```python
from build123d import *

# Parameters (mm, degrees)
SKETCH1_W          = 58
SKETCH1_H          = 34
EXTRUDE1_DEPTH     = 1.6
SKETCH2_W          = 38
SKETCH2_H          = 6
EXTRUDE2_DEPTH     = 8.5
SKETCH3_W          = 9
SKETCH3_H          = 33
EXTRUDE3_DEPTH     = 9.2
SKETCH4_W          = 16.4
SKETCH4_H          = 12.2
EXTRUDE4_DEPTH     = 11
CUT_EXTRUDE1_DEPTH = 14
FILLET1_R          = 1
FILLET2_R          = 0.5


with BuildPart() as part:
    # Sketch1 → Extrude1 (new body)
    with BuildSketch(Plane.XY):
        with Locations((29, 17)):
            Rectangle(SKETCH1_W, SKETCH1_H)
    extrude(amount=EXTRUDE1_DEPTH)

    # Sketch2 → Extrude2 (add)
    with BuildSketch(Plane(origin=(0, 0, 0), x_dir=(-1, 0, 0), z_dir=(0, 0, -1))):
        with Locations((-29, 30)):
            Rectangle(SKETCH2_W, SKETCH2_H)
        with Locations((-29, 4)):
            Rectangle(SKETCH2_W, SKETCH2_H)
    extrude(amount=EXTRUDE2_DEPTH)

    # Sketch3 → Extrude3 (add)
    with BuildSketch(Plane.XY.offset(1.6)):
        with Locations((53, 17)):
            Rectangle(SKETCH3_W, SKETCH3_H)
    extrude(amount=EXTRUDE3_DEPTH)

    # Sketch4 → Extrude4 (add)
    with BuildSketch(Plane.XY.offset(1.6)):
        with Locations((1.8, 17)):
            Rectangle(SKETCH4_W, SKETCH4_H)
    extrude(amount=EXTRUDE4_DEPTH)

    # Sketch5 → Cut-Extrude1 (cut)
    with BuildSketch(Plane.ZY.offset(6.4)):
        Polygon((8.8, 21.3), (10.8, 19.3), (10.8, 14.7), (8.8, 12.7), (3.4, 12.7), (3.4, 21.3), align=None)
    extrude(amount=-CUT_EXTRUDE1_DEPTH, mode=Mode.SUBTRACT)

    # Fillet1
    fillet1_edges = [part.edges().sort_by_distance(p)[0] for p in [
        (-3.2, 23.1, 1.6),
        (-3.2, 10.9, 1.6),
        (1.8, 23.1, 12.6),
        (1.8, 10.9, 12.6),
    ]]
    fillet(fillet1_edges, radius=FILLET1_R)

    # Fillet2
    fillet2_edges = [part.edges().sort_by_distance(p)[0] for p in [
        (-6.4, 21.3, 6.1),
        (-6.4, 17, 3.4),
        (-6.4, 12.7, 6.1),
        (-6.4, 13.7, 9.8),
        (-6.4, 17, 10.8),
        (-6.4, 20.3, 9.8),
        (-6.4, 17, 12.6),
        (-6.4, 10.9, 7.1),
        (-6.4, 17, 1.6),
        (-6.4, 23.1, 7.1),
        (-6.4, 22.807106781, 12.307106781),
        (-6.4, 22.807106781, 1.892893219),
        (-6.4, 11.192893219, 1.892893219),
        (-6.4, 11.192893219, 12.307106781),
    ]]
    fillet(fillet2_edges, radius=FILLET2_R)


solid = part.part
```
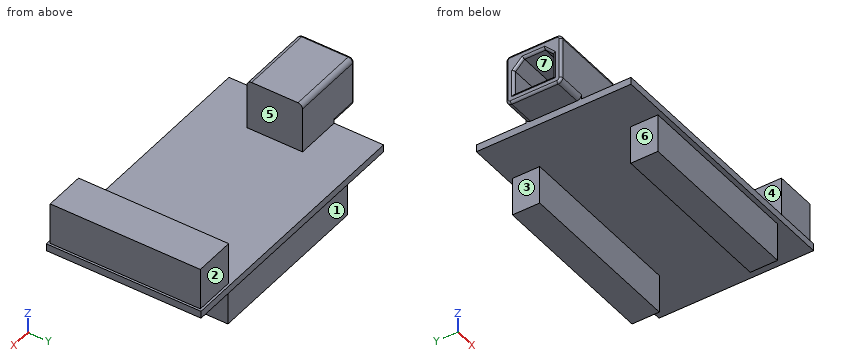
Model file for the job. Use its own axes, mm. Face numbers are marked on the shaded views. A direction names the side the tool comes from. Give positions to 0.01 mm unless a question says otherwise; leave off trailing zeros. Loops run counter-clockwise (first coordinate to the right, second up) from the corner with the lowest first, then second, coordinate; pieces in that order, holes last. Notation, with made-up numbers: (49, 70) -> (97, 70) arc R32 cw to (97, 105) -> close; hole circle Ø1 at (89, -27.5). An arc over 180 degrees is marked (long way). Use CSV: the item, a comma, the result in double quotes. Start each with the question number.
1) Slice it at D-D on x = 9. Give the cut face in (y, z), plus the area to 3 significant figures.
2) Wall check: line 1 (X direction, y = 15, z = 4.75); line 2 (Y direction, x = 30, z = -5.75); line 3 (X direction, y = 17, z = 11.75). Give the ranges that are in metal, low to high.
3) Slice it at C-C on y = 30. Give the cut face in (x, z), plus the area to 3 significant figures.
4) Mould opens along X. For the marked faces 5, 6 and 7 say: released by +X, released by -X, zero draft, split by the parting line, or undercut.
5) Tool access for the marked faces 1, 2, 3 and 4: list every direction of +Z, -Z, +X, -X, +Y, -Y with a clear straight run to the whole face (end or side of a thin tool).
6) Slice it at B-B on x = 1. Give the cut face in (y, z), plus the area to 3 significant figures.
7) Slice it at A-A on z = -5. Give the cut face in (x, y).
8) Flat gauge pins, fed straight in: pin 1 Ø8 at (x, y) = (6, 15) entering from -Z; pin 2 Ø2.5 at (x, z) = (35, -5) entering from +Y; pin 3 Ø4 at (x, z) = (1.5, 6.5) entering from +Y. Where does each tip first touch, or does it go through?
Computed values:
1,outline,"(0, 0) -> (34, 0) -> (34, 1.6) -> (23.1, 1.6) -> (23.1, 11.6) arc R1 ccw to (22.1, 12.6) -> (11.9, 12.6) arc R1 ccw to (10.9, 11.6) -> (10.9, 1.6) -> (0, 1.6) -> close"
1,area,"188 mm^2"
2,line 1,"x = 7.6 to 10, 48.5 to 57.5"
2,line 2,"y = 1 to 7, 27 to 33"
2,line 3,"x = -6.4 to 10"
3,outline,"(0, 0) -> (10, 0) -> (10, -8.5) -> (48, -8.5) -> (48, 0) -> (58, 0) -> (58, 1.6) -> (57.5, 1.6) -> (57.5, 10.8) -> (48.5, 10.8) -> (48.5, 1.6) -> (0, 1.6) -> close"
3,area,"499 mm^2"
4,face 5,"undercut"
4,face 6,"released by -X"
4,face 7,"zero draft"
5,face 1,"-Z, +X, -X, +Y"
5,face 2,"+Z, +X, -X, +Y"
5,face 3,"-Z, -X, +Y, -Y"
5,face 4,"+Z, +Y, -Y"
6,outline,"(0, 0) -> (34, 0) -> (34, 1.6) -> (23.1, 1.6) -> (23.1, 11.6) arc R1 ccw to (22.1, 12.6) -> (11.9, 12.6) arc R1 ccw to (10.9, 11.6) -> (10.9, 1.6) -> (0, 1.6) -> close; hole (12.7, 3.4) -> (21.3, 3.4) -> (21.3, 8.8) -> (19.3, 10.8) -> (14.7, 10.8) -> (12.7, 8.8) -> close"
6,area,"129 mm^2"
7,outline,"(10, 1) -> (48, 1) -> (48, 7) -> (10, 7) -> close; (10, 27) -> (48, 27) -> (48, 33) -> (10, 33) -> close"
8,pin 1,"stops at z = 0"
8,pin 2,"stops at y = 33"
8,pin 3,"stops at y = 23.1"
